Here's how the part is built. I have some questions about the finished solid (model axes, mm). A direction names the side the tool comes from. Give positions to 0.01 mm unless a question says otherwise; leave off trailing zeros. Write each loop counter-clockwise with the first axis right and the second up, starting at its lowest first coordinate (ties: lowest second). Pieces come first, ordered by that corner, then holes. Notation, with made-up numbers: (-37, 30) -> (15, 30) arc R21 ccw to (15, 55) -> close; hole circle Ø9 at (87.25, 70). An arc over 180 degrees is marked (long way). Return JSON: item names as keys, results as strings.
from build123d import *

# Parameters (mm, degrees)
CHAMFER1_SIZE = 1
FILLET1_R     = 0.6
CHAMFER3_SIZE = 1
CHAMFER4_SIZE = 0.5


with BuildPart() as part:
    # Sketch1 → Revolve1 (revolve)
    with BuildSketch(Plane.XY, mode=Mode.PRIVATE) as revolve1_sk:
        Polygon((0, 0), (0, 12.5), (8, 12.5), (8, 8), (13, 8), (13, 6), (46, 6), (46, 4.076239569), (47.4, 4.076239569), (49, 5), (58, 5), (58, 0), align=None)
    revolve(revolve1_sk.sketch.rotate(Axis((-9.676136096, 0, 0), (1, 0, 0)), 90), axis=Axis((-9.676136096, 0, 0), (1, 0, 0)))

    # Chamfer1
    chamfer1_edges = [part.edges().sort_by_distance(p)[0] for p in [
        (46, 0, -6),
        (8, 0, -12.5),
        (0, 0, -12.5),
    ]]
    chamfer(chamfer1_edges, length=CHAMFER1_SIZE)

    # Fillet1
    fillet1_edges = [part.edges().sort_by_distance(p)[0] for p in [
        (47.4, 0, -4.076239569),
        (46, 0, -4.076239569),
    ]]
    fillet(fillet1_edges, radius=FILLET1_R)

    # Chamfer3
    chamfer3_edges = [part.edges().sort_by_distance(p)[0] for p in [
        (58, 0, -5),
    ]]
    chamfer(chamfer3_edges, length=CHAMFER3_SIZE)

    # Chamfer4
    chamfer4_edges = [part.edges().sort_by_distance(p)[0] for p in [
        (13, 0, -8),
    ]]
    chamfer(chamfer4_edges, length=CHAMFER4_SIZE)


solid = part.part
1. If I drill on line 1 (Z direction, x = 52, y = -1.75); line 2 (X direction, y = -8, z = 1.25); line 3 (X direction, y = -5.75, z = -3), over which ranges is the centre line in solid material (lowest first)? Write a range as [from, to].
Taken from the geometry:
{"line 1": "z = [-4.68, 4.68]", "line 2": "x = [0, 8]", "line 3": "x = [0, 13]"}
2. Which directions (+Z, -Z, +X, -X, +Y, -Y) give clear straight access to the entire face, cutting with the end or side of a thin tool? Please do faces 4 (the face through (29.224, -1.802, 5.723)), 5 (the face through (0, 0, 0)).
Taken from the geometry:
{"face 4": "+X", "face 5": "+Z, -Z, -X, +Y, -Y"}
3. For pin 1 Ø12 at (x, z) = (45.5, 0) entering from +Y; pin 2 Ø1.5 at (x, y) = (10, -4) entering from -Z; pin 3 Ø12 at (x, y) = (40.5, 5.5) entering from -Z, each with a flat end and sliding along its axis, tell me the tip position at first contact or that it passes through.
Taken from the geometry:
{"pin 1": "stops at y = 6", "pin 2": "stops at z = -7.31", "pin 3": "stops at z = -6"}
4. Suppose I cut it at A-A, the plane x = 54. List the corners of the cut face in (y, z) for me.
Taken from the geometry:
{"outline": "circle Ø10 at (0, 0)"}
5. If we mould it in two halves opening along X, with no side actions, what happens to faces 1 (the face through (53, 0, -5)), 2 (the face through (46.924, 3.616, 1.881)), 3 (the face through (13, -6, 2))? For each: released by +X, released by -X, zero draft, split by the parting line, or undercut.
Taken from the geometry:
{"face 1": "zero draft", "face 2": "undercut", "face 3": "released by +X"}
6. Suppose I cut it at B-B, the plane x = 14. List the corners of the cut face in (y, z) for me, and give its area (3 significant figures).
Taken from the geometry:
{"outline": "circle Ø12 at (0, 0)", "area": "113 mm²"}
